```python
from build123d import *

# Parameters (mm, degrees)
F0_R     = 2.5
F0_R_2   = 1.4107797467
F0_W     = 10
F0_H     = 2
F1_DEPTH = 2
F2_DEPTH = 4
F3_DEPTH = 7


# Not quite as in the source:
# - a fillet or chamfer that OpenCascade refuses, or shapes differently, is made with other operations: its cross-section is extruded or revolved along the edge and cut away or added


with BuildPart() as f1:
    # F0 (on Top) → F1 (new body)
    with BuildSketch(Plane.XY):
        Polygon((19, -18), (19, -16), (10.7328139991, -16), (-31, -16), (-31, 16), (31, 16), (31, -16), (29, -16), (29, -18), (33, -18), (33, 18), (-33, 18), (-33, -18), align=None)
        Polygon((-30, -15), (-30, 15), (-26.5, 15), (30, 15), (30, -15), (29, -15), (29, -16), (31, -16), (31, 16), (-31, 16), (-31, -16), (10.7328139991, -16), (19, -16), (19, -15), align=None)
        Polygon((-26.5, 15), (-30, 15), (-30, -15), (19, -15), (24, -15), (29, -15), (30, -15), (30, 15), align=None)
        with Locations((-26.5, -11.5)):
            Circle(F0_R, mode=Mode.SUBTRACT)
        with Locations((26.5, -11.5)):
            Circle(F0_R, mode=Mode.SUBTRACT)
        with BuildLine():
            ThreePointArc((-24, 11.5), (-28.267766953, 9.732233047), (-26.5, 14))
            ThreePointArc((-26.5, 14), (-24.732233047, 13.267766953), (-24, 11.5))
        make_face(mode=Mode.SUBTRACT)
        with Locations((26.5, 11.5)):
            Circle(F0_R, mode=Mode.SUBTRACT)
        with BuildLine():
            ThreePointArc((-24, 11.5), (-24.732233047, 13.267766953), (-26.5, 14))
            ThreePointArc((-26.5, 14), (-28.267766953, 9.732233047), (-24, 11.5))
        make_face()
        with BuildLine():
            ThreePointArc((-25.0892202533, 11.5), (-27.4975719256, 10.5024280744), (-26.5, 12.9107797467))
            ThreePointArc((-26.5, 12.9107797467), (-25.5024280744, 12.4975719256), (-25.0892202533, 11.5))
        make_face(mode=Mode.SUBTRACT)
        with Locations((-26.5, -11.5)):
            Circle(F0_R)
        with Locations((-26.5, -11.5)):
            Circle(F0_R_2, mode=Mode.SUBTRACT)
        with Locations((26.5, -11.5)):
            Circle(F0_R)
        with Locations((26.5, -11.5)):
            Circle(F0_R_2, mode=Mode.SUBTRACT)
        with Locations((26.5, 11.5)):
            Circle(F0_R)
        with Locations((26.5, 11.5)):
            Circle(F0_R_2, mode=Mode.SUBTRACT)
        Polygon((24, -15), (19, -15), (19, -16), (29, -16), (29, -15), align=None)
        with Locations((24, -17)):
            Rectangle(F0_W, F0_H)
    extrude(amount=F1_DEPTH)

    # F0 (on Top) → F2 (join)
    with BuildSketch(Plane.XY):
        with Locations((-26.5, -11.5)):
            Circle(F0_R)
        with Locations((-26.5, -11.5)):
            Circle(F0_R_2, mode=Mode.SUBTRACT)
        with BuildLine():
            ThreePointArc((-24, 11.5), (-24.732233047, 13.267766953), (-26.5, 14))
            ThreePointArc((-26.5, 14), (-28.267766953, 9.732233047), (-24, 11.5))
        make_face()
        with BuildLine():
            ThreePointArc((-25.0892202533, 11.5), (-27.4975719256, 10.5024280744), (-26.5, 12.9107797467))
            ThreePointArc((-26.5, 12.9107797467), (-25.5024280744, 12.4975719256), (-25.0892202533, 11.5))
        make_face(mode=Mode.SUBTRACT)
        with Locations((26.5, -11.5)):
            Circle(F0_R)
        with Locations((26.5, -11.5)):
            Circle(F0_R_2, mode=Mode.SUBTRACT)
        with Locations((26.5, 11.5)):
            Circle(F0_R)
        with Locations((26.5, 11.5)):
            Circle(F0_R_2, mode=Mode.SUBTRACT)
    extrude(amount=F2_DEPTH)

    # F0 (on Top) → F3 (join)
    with BuildSketch(Plane.XY):
        Polygon((19, -18), (19, -16), (10.7328139991, -16), (-31, -16), (-31, 16), (31, 16), (31, -16), (29, -16), (29, -18), (33, -18), (33, 18), (-33, 18), (-33, -18), align=None)
    extrude(amount=F3_DEPTH)

    # F4: chamfer of 1.5 on 4 edges, made by hand

    # F4_s1 → F4_t2 (revolve, cut)
    with BuildSketch(Plane.XZ.offset(11.5)):
        with BuildLine():
            Line((29.4532061535, -0.0424264069), (27.8683533398, 1.5424264069))
            Line((27.8683533398, 1.5424264069), (27.8383533398, 1.5424264069))
            ThreePointArc((27.8383533398, 1.5424264069), (27.8807797467, 0.7712132034), (27.8807797467, 0))
            Line((27.8807797467, 0), (27.9107797467, -0.03))
            ThreePointArc((27.9107797467, -0.03), (28.6819929501, -0.03), (29.4532061535, -0.0724264069))
            Line((29.4532061535, -0.0724264069), (29.4532061535, -0.0424264069))
        make_face()
    revolve(axis=Axis((26.5, -11.5, 0), (0, 0, 1)), mode=Mode.SUBTRACT)

    # F4_s3 → F4_t4 (revolve, cut)
    with BuildSketch(Plane.XZ.offset(-11.5)):
        with BuildLine():
            Line((29.4532061535, -0.0424264069), (27.8683533398, 1.5424264069))
            Line((27.8683533398, 1.5424264069), (27.8383533398, 1.5424264069))
            ThreePointArc((27.8383533398, 1.5424264069), (27.8807797467, 0.7712132034), (27.8807797467, 0))
            Line((27.8807797467, 0), (27.9107797467, -0.03))
            ThreePointArc((27.9107797467, -0.03), (28.6819929501, -0.03), (29.4532061535, -0.0724264069))
            Line((29.4532061535, -0.0724264069), (29.4532061535, -0.0424264069))
        make_face()
    revolve(axis=Axis((26.5, 11.5, 0), (0, 0, 1)), mode=Mode.SUBTRACT)

    # F4_s5 → F4_t6 (revolve, cut)
    with BuildSketch(Plane.XZ.offset(-11.5)):
        with BuildLine():
            Line((-23.5467938465, -0.0424264069), (-25.1316466602, 1.5424264069))
            Line((-25.1316466602, 1.5424264069), (-25.1616466602, 1.5424264069))
            ThreePointArc((-25.1616466602, 1.5424264069), (-25.1192202533, 0.7712132034), (-25.1192202533, 0))
            Line((-25.1192202533, 0), (-25.0892202533, -0.03))
            ThreePointArc((-25.0892202533, -0.03), (-24.3180070499, -0.03), (-23.5467938465, -0.0724264069))
            Line((-23.5467938465, -0.0724264069), (-23.5467938465, -0.0424264069))
        make_face()
    revolve(axis=Axis((-26.5, 11.5, 0), (0, 0, 1)), mode=Mode.SUBTRACT)

    # F4_s7 → F4_t8 (revolve, cut)
    with BuildSketch(Plane.XZ.offset(11.5)):
        with BuildLine():
            Line((-23.5467938465, -0.0424264069), (-25.1316466602, 1.5424264069))
            Line((-25.1316466602, 1.5424264069), (-25.1616466602, 1.5424264069))
            ThreePointArc((-25.1616466602, 1.5424264069), (-25.1192202533, 0.7712132034), (-25.1192202533, 0))
            Line((-25.1192202533, 0), (-25.0892202533, -0.03))
            ThreePointArc((-25.0892202533, -0.03), (-24.3180070499, -0.03), (-23.5467938465, -0.0724264069))
            Line((-23.5467938465, -0.0724264069), (-23.5467938465, -0.0424264069))
        make_face()
    revolve(axis=Axis((-26.5, -11.5, 0), (0, 0, 1)), mode=Mode.SUBTRACT)


solid = f1.part
```
Could you check a few things on this model? Use its own coordinates, in mm. A direction names the side the tool comes from. Round coordinates to 2 decimals unless told otherwise and drop trailing zeros. Loops run counter-clockwise (first coordinate to the right, second up) from the corner with the lowest first, then second, coordinate; pieces in that order, holes last.
Q1. I want a section at B-B (y = -11.5). Write out the boundary of the cut face in (x, z), and give its area (3 significant figures).
Q2. I want a section at D-D (y = -3). Write out the boundary of the cut face in (x, z), and give its area (3 significant figures).
Q3. I want a section at A-A (x = 26.5). Write out the boundary of the cut face in (y, z).
Q4. I want a section at C-C (z = 6.25). Write out the boundary of the cut face in (x, y).
Q5. Thinking about a two-plate mould opening in Y: for faces 4 (the flat face through (0, 18, 3)), 5 (the flat face through (-6, -16, 4)), 6 (the flat face through (19, -17, 4)), which applies, pulls with the +Y half, pulls with the -Y half, needs draft (parallel to the pull), parting line crosses it, or undercut?
Q6. On a 3-axis mill with a long thin cutter (end or side, diameter ignored), from which of +Z, -Z, +X, -X, +Y, -Y can I reach the whole of each face in a straight line? I mean faces 1 (the flat face through (28, -13, 4)), 2 (the cylindrical face through (25.38, 10.64, 2.73)), 3 (the flat face through (31, 0, 4)). Say none if no direction works.
Q7. For P1, Ø5.5, axis at x = 27.5, y = 11, coming from the +Z side; P2, Ø1.5, axis at x = 26, z = 6, coming from the -Y side; P3, Ø5, axis at x = 12.5, y = -2.5, coming from the +Z side, each with a flat end and sliding along its axis, tell me the tip position at first contact or that it passes through.
Q8. Please list where these lines run through material, in increasing order: L1, parallel to X at y = 11.5, z = 2.85; L2, parallel to Y at x = 26.5, z = 2.05; L3, parallel to Y at x = -6, z = 3.25.
Answer below:
1. outline: (-33, 0) - (-29.41, 0) - (-27.91, 1.5) - (-27.91, 4) - (-29, 4) - (-29, 2) - (-31, 2) - (-31, 7) - (-33, 7) - close; (-25.09, 1.5) - (-23.59, 0) - (23.59, 0) - (25.09, 1.5) - (25.09, 4) - (24, 4) - (24, 2) - (-24, 2) - (-24, 4) - (-25.09, 4) - close; (27.91, 1.5) - (29.41, 0) - (33, 0) - (33, 7) - (31, 7) - (31, 2) - (29, 2) - (29, 4) - (27.91, 4) - close
1. area: 145 mm2
2. outline: (-33, 0) - (33, 0) - (33, 7) - (31, 7) - (31, 2) - (-31, 2) - (-31, 7) - (-33, 7) - close
2. area: 152 mm2
3. outline: (-18, 0) - (-14.41, 0) - (-12.91, 1.5) - (-12.91, 4) - (-14, 4) - (-14, 2) - (-18, 2) - close; (-10.09, 1.5) - (-8.59, 0) - (8.59, 0) - (10.09, 1.5) - (10.09, 4) - (9, 4) - (9, 2) - (-9, 2) - (-9, 4) - (-10.09, 4) - close; (12.91, 1.5) - (14.41, 0) - (18, 0) - (18, 7) - (16, 7) - (16, 2) - (14, 2) - (14, 4) - (12.91, 4) - close
4. outline: (-33, -18) - (19, -18) - (19, -16) - (-31, -16) - (-31, 16) - (31, 16) - (31, -16) - (29, -16) - (29, -18) - (33, -18) - (33, 18) - (-33, 18) - close
5. face 4: pulls with the +Y half
5. face 5: undercut
5. face 6: needs draft
6. face 1: +Z, -Y
6. face 2: +Z, -Z
6. face 3: +Z
7. P1: stops at z = 4
7. P2: stops at y = 16
7. P3: stops at z = 2
8. L1: x = -33 to -31, -29 to -27.91, -25.09 to -24, 24 to 25.09, 27.91 to 29, 31 to 33
8. L2: y = -14 to -12.91, -10.09 to -9, 9 to 10.09, 12.91 to 14, 16 to 18
8. L3: y = -18 to -16, 16 to 18
